```python
from build123d import *

# Parameters (mm, degrees)
F0_W     = 70
F0_H     = 40
F1_DEPTH = 60
F2_W     = 40
F2_H     = 30
F3_DEPTH = 50
F4_W     = 59
F4_H     = 29
F5_DEPTH = 2.5


with BuildPart() as f1:
    # F0 (on Right) → F1 (new body)
    with BuildSketch(Plane.YZ):
        with Locations((35, 20)):
            Rectangle(F0_W, F0_H)
    extrude(amount=F1_DEPTH)

    # F2 (on face) → F3 (cut)
    with BuildSketch(Plane.YZ.offset(60)):
        with Locations((35, 20)):
            Rectangle(F2_W, F2_H)
    extrude(amount=-F3_DEPTH, mode=Mode.SUBTRACT)

    # F4 (on face) → F5 (join)
    with BuildSketch(Plane(origin=(0, 0, 0), x_dir=(0, -1, 0), z_dir=(-1, 0, 0))):
        with Locations((-35, 20)):
            Rectangle(F4_W, F4_H)
    extrude(amount=F5_DEPTH)


solid = f1.part
```
Source: CAD feature listing. Evaluate the final solid. Frame: model axes, mm. A direction names the side the tool comes from. Coordinates: 2 decimals unless noted, no trailing zeros. Loops run counter-clockwise (first coordinate to the right, second up) from the corner with the lowest first, then second, coordinate; pieces in that order, holes last. Notation, with made-up numbers: M 65,20 L 92,20 A18 ccw 92,49 Z; hole C -18,83 d10. An arc over 180 degrees is marked long. Use a Markdown table: item, result. Add a question column.
Q1. Section query C-C, the plane y = 33.5. Return loops of the section in (x, z), and give its area (4 significant figures).
Q2. Section query B-B, the plane z = 25.5. Return loops of the section in (x, y).
Q3. Draft query along Y for faces 6 (the flat face through (10, 35, 20)), 7 (the flat face through (30, 70, 20)), 8 (the flat face through (30, 0, 20)), 9 (the flat face through (35, 15, 20)). Return one class per face: pulls with the +Y half, pulls with the -Y half, needs draft (parallel to the pull), parting line crosses it, or undercut.
Q4. Access query for faces 1 (the flat face through (-1, 64.5, 20)), 2 (the flat face through (35, 35, 5)), 3 (the flat face through (-1, 5.5, 20)), 4 (the flat face through (-1, 35, 34.5)), 5 (the flat face through (-1, 35, 5.5)). Directions: +Z, -Z, +X, -X, +Y, -Y. A direction counts if a zero-diameter tool reaches every point of the face in a straight line with its end or side. Return the directions, or none.
Q5. First-contact query: pin 1 (3 mm diameter, centred on x = -0.5, z = 22, fed in from +Y); pin 2 (1.2 mm diameter, centred on x = -1, y = 30.5, fed in from +Z); pin 3 (2 mm diameter, centred on x = -1.5, y = 30.5, fed in from -Z); pin 4 (1.2 mm diameter, centred on x = -1, z = 24.5, fed in from -Y). Flat tips, straight axial feed; report the tip coordinate or a pass-through.
Q6. Section query D-D, the plane y = 66.5. Return loops of the section in (x, z), and give its area (3 significant figures).
Q7. Material intervals for L1, parallel to Z at x = 45.5, y = 53; L2, parallel to Y at x = 41, z = 27; L3, parallel to X at y = 40, z = 12, sorted ascending.
Q8. Section query A-A, the plane x = 20. Return loops of the section in (y, z), and give its area (3 significant figures).
Result:
| question | item | result |
|---|---|---|
| 1 | outline | M -2.5,5.5 L 0,5.5 L 0,0 L 60,0 L 60,5 L 10,5 L 10,35 L 60,35 L 60,40 L 0,40 L 0,34.5 L -2.5,34.5 Z |
| 1 | area | 972.5 mm2 |
| 2 | outline | M -2.5,5.5 L 0,5.5 L 0,0 L 60,0 L 60,15 L 10,15 L 10,55 L 60,55 L 60,70 L 0,70 L 0,64.5 L -2.5,64.5 Z |
| 3 | face 6 | undercut |
| 3 | face 7 | pulls with the +Y half |
| 3 | face 8 | pulls with the -Y half |
| 3 | face 9 | undercut |
| 4 | face 1 | +Z, -Z, -X, +Y |
| 4 | face 2 | +X |
| 4 | face 3 | +Z, -Z, -X, -Y |
| 4 | face 4 | +Z, -X, +Y, -Y |
| 4 | face 5 | -Z, -X, +Y, -Y |
| 5 | pin 1 | stops at y = 70 |
| 5 | pin 2 | stops at z = 34.5 |
| 5 | pin 3 | stops at z = 5.5 |
| 5 | pin 4 | stops at y = 5.5 |
| 6 | outline | M 0,0 L 60,0 L 60,40 L 0,40 Z |
| 6 | area | 2,400 mm2 |
| 7 | L1 | z = 0 to 5, 35 to 40 |
| 7 | L2 | y = 0 to 15, 55 to 70 |
| 7 | L3 | x = -2.5 to 10 |
| 8 | outline | M 0,0 L 70,0 L 70,40 L 0,40 Z; hole M 15,5 L 55,5 L 55,35 L 15,35 Z |
| 8 | area | 1,600 mm2 |
